For this review, take the finished solid that the model builds, in its own axes (mm). Face numbers are marked on the shaded views. A direction names the side the tool comes from. Give positions to 0.01 mm unless a question says otherwise; leave off trailing zeros. Order: outer loops, then holes, each group sorted by start corner. A loop starts at its lowest first (then second) coordinate and runs counter-clockwise, first axis right, second up.
Item 1: Consider section B-B (z = 28.03). Give the boundary of the cut face in (x, y), plus the area to 3 significant figures.
Item 2: The part is to be moulded in two halves that separate along X. For the marked faces 1, 2 and 3, say which applies: released by +X, released by -X, zero draft, split by the parting line, or undercut.
Item 3: For probe 1 along X at (y, z) = (22, -1); probe 2 along X at (y, z) = (29.45, -28.03); probe 3 along Y at (x, z) = (65, -21.5), list the stretches that pass through material, from the lowest coordinate up.
Item 4: For P1, Ø8, axis at x = 50, y = 24.5, coming from the -Z side; P2, Ø3, axis at x = 160.22, z = -15.57, coming from the +Y side; P3, Ø12, axis at x = 166, z = 5, coming from the +Y side; P4, Ø3, axis at x = -41.22, z = 0, coming from the +Y side, all flat-tipped, find the tip position at first contact; note any pin that passes through.
Item 5: Machinability: for the marked faces 4, 5 and 6, which of the approach directions +Z, -Z, +X, -X, +Y, -Y give a long, thin tool a straight path to every point of the face, cutting with its end or side? Answer none if there is none.
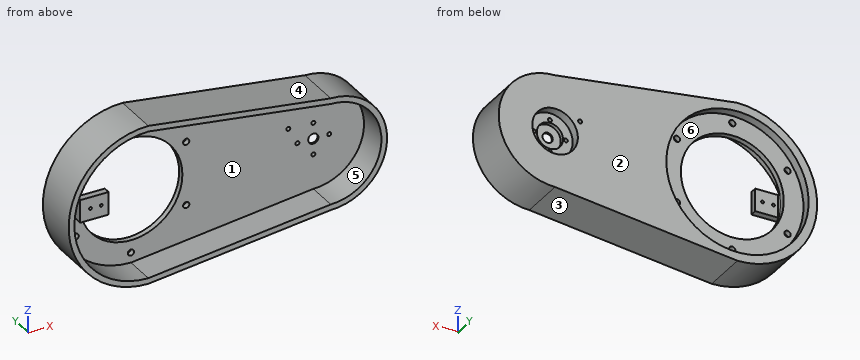
```python
from build123d import *

# Parameters (mm, degrees)
BOSS_EXTRUDE1_DEPTH = 40
SKETCH2_R           = 45.22
SKETCH2_R_2         = 2.75
CUT_EXTRUDE1_DEPTH  = 28
SKETCH4_R           = 62.5
CUT_EXTRUDE2_DEPTH  = 8
CUT_EXTRUDE3_DEPTH  = 27
SKETCH6_R           = 4.5
SKETCH6_R_2         = 1.75
CUT_EXTRUDE4_DEPTH  = 23
SKETCH6_3_R         = 11.5
SKETCH6_3_R_2       = 4.5
CUT_EXTRUDE5_DEPTH  = 11.5
BOSS_EXTRUDE2_DEPTH = 10
SKETCH8_W           = 20
SKETCH8_H           = 6
BOSS_EXTRUDE3_DEPTH = 20
SKETCH9_R           = 1.25
CUT_EXTRUDE6_DEPTH  = 20
SKETCH6_4_R         = 20
CUT_EXTRUDE7_DEPTH  = 8
SKETCH11_R          = 4.5
SKETCH11_R_2        = 1.75
CUT_EXTRUDE8_DEPTH  = 168


with BuildPart() as part:
    # Sketch1 → Boss-Extrude1 (new body)
    with BuildSketch(Plane(origin=(0, 0, 0), x_dir=(1, 0, 0), z_dir=(0, 1, 0))):
        with BuildLine():
            Line((0, 70), (160.2226, 51.102080384))
            ThreePointArc((160.2226, 51.102080384), (209.74985375, 1.574826635), (160.2226, -47.952427115))
            Line((160.2226, -47.952427115), (0, -70))
            ThreePointArc((0, -70), (-70, 0), (0, 70))
        make_face()
    extrude(amount=BOSS_EXTRUDE1_DEPTH)

    # Sketch2 → Cut-Extrude1 (cut)
    with BuildSketch(Plane(origin=(0, 40, 0), x_dir=(1, 0, 0), z_dir=(0, 1, 0))):
        Circle(SKETCH2_R)
        with Locations((0, 56.06)):
            Circle(SKETCH2_R_2)
        with Locations((-48.549384136, 28.03)):
            Circle(SKETCH2_R_2)
        with Locations((-48.549384136, -28.03)):
            Circle(SKETCH2_R_2)
        with Locations((0, -56.06)):
            Circle(SKETCH2_R_2)
        with Locations((48.549384136, -28.03)):
            Circle(SKETCH2_R_2)
        with Locations((48.549384136, 28.03)):
            Circle(SKETCH2_R_2)
    extrude(amount=-CUT_EXTRUDE1_DEPTH, mode=Mode.SUBTRACT)

    # Sketch4 → Cut-Extrude2 (cut)
    with BuildSketch(Plane(origin=(0, 40, 0), x_dir=(1, 0, 0), z_dir=(0, 1, 0))):
        Circle(SKETCH4_R)
    extrude(amount=-CUT_EXTRUDE2_DEPTH, mode=Mode.SUBTRACT)

    # Sketch5 → Cut-Extrude3 (cut)
    with BuildSketch(Plane.XZ):
        with BuildLine():
            Line((160.2226, 42.955173365), (0, 65))
            ThreePointArc((0, 65), (-65, 0), (0, -65))
            Line((0, -65), (160.2226, -46.104826635))
            ThreePointArc((160.2226, -46.104826635), (204.7526, -1.574826635), (160.2226, 42.955173365))
        make_face()
    extrude(amount=-CUT_EXTRUDE3_DEPTH, mode=Mode.SUBTRACT)

    # Sketch6 → Cut-Extrude4 (cut)
    with BuildSketch(Plane(origin=(0, 40, 0), x_dir=(1, 0, 0), z_dir=(0, 1, 0))):
        with Locations((160.2226, 1.574826635)):
            Circle(SKETCH6_R)
        with Locations((160.2226, -12.425173365)):
            Circle(SKETCH6_R_2)
        with Locations((174.2226, 1.574826635)):
            Circle(SKETCH6_R_2)
        with Locations((160.2226, 15.574826635)):
            Circle(SKETCH6_R_2)
        with Locations((146.2226, 1.574826635)):
            Circle(SKETCH6_R_2)
    extrude(amount=-CUT_EXTRUDE4_DEPTH, mode=Mode.SUBTRACT)

    # Sketch6_3 → Cut-Extrude5 (cut)
    with BuildSketch(Plane(origin=(0, 40, 0), x_dir=(1, 0, 0), z_dir=(0, 1, 0))):
        with Locations((160.2226, 1.574826635)):
            Circle(SKETCH6_3_R)
        with Locations((160.2226, 1.574826635)):
            Circle(SKETCH6_3_R_2, mode=Mode.SUBTRACT)
    extrude(amount=-CUT_EXTRUDE5_DEPTH, mode=Mode.SUBTRACT)

    # Sketch7 → Boss-Extrude2 (add)
    with BuildSketch(Plane.XZ.offset(-27)):
        Polygon((-45.22, 0), (-45.22, 10), (-50.22, 10), (-50.22, -10), (-45.22, -10), align=None)
    extrude(amount=BOSS_EXTRUDE2_DEPTH)

    # Sketch8 → Boss-Extrude3 (add)
    with BuildSketch(Plane(origin=(-45.22, 0, 0), x_dir=(0, 0, -1), z_dir=(1, 0, 0))):
        with Locations((0, 20)):
            Rectangle(SKETCH8_W, SKETCH8_H)
    extrude(amount=BOSS_EXTRUDE3_DEPTH)

    # Sketch9 → Cut-Extrude6 (cut)
    with BuildSketch(Plane.XZ.offset(-17)):
        with Locations((-31.72, 0)):
            Circle(SKETCH9_R)
        with Locations((-41.22, 0)):
            Circle(SKETCH9_R)
    extrude(amount=-CUT_EXTRUDE6_DEPTH, mode=Mode.SUBTRACT)

    # Sketch6_4 → Cut-Extrude7 (cut)
    with BuildSketch(Plane(origin=(0, 40, 0), x_dir=(1, 0, 0), z_dir=(0, 1, 0))):
        with Locations((160.2226, 1.574826635)):
            Circle(SKETCH6_4_R)
    extrude(amount=-CUT_EXTRUDE7_DEPTH, mode=Mode.SUBTRACT)

    # Sketch11 → Cut-Extrude8 (cut)
    with BuildSketch(Plane.XZ.offset(-27)):
        with Locations((160.2226, -1.574826635)):
            Circle(SKETCH11_R)
        with Locations((138.2226, 13.425173365)):
            Circle(SKETCH11_R_2)
    extrude(amount=-CUT_EXTRUDE8_DEPTH, mode=Mode.SUBTRACT)


solid = part.part
```
Resolved:
1. outline: (-64.14, 0) - (-58.65, 0) - (-58.65, 27) - (-51.3, 27) - (-51.3, 32) - (-55.86, 32) - (-55.86, 40) - (-64.14, 40) - close; (-45.8, 27) - (-35.48, 27) - (-35.48, 32) - (-45.8, 32) - close; (35.48, 27) - (45.8, 27) - (45.8, 32) - (35.48, 32) - close; (51.3, 27) - (193.49, 27) - (193.49, 0) - (199.93, 0) - (199.93, 40) - (55.86, 40) - (55.86, 32) - (51.3, 32) - close
1. area: 2,450 mm2
2. face 1: undercut
2. face 2: zero draft
2. face 3: released by +X
3. probe 1: x = -69.99 to -64.99, -50.22 to -41.97, -40.47 to -32.47, -30.97 to -25.22, 204.75 to 209.75
3. probe 2: x = -64.14 to -51.3, -45.8 to -35.48, 35.48 to 45.8, 51.3 to 202.09
3. probe 3: y = 27 to 40
4. P1: stops at z = -64.57
4. P2: passes through
4. P3: stops at y = 32
4. P4: stops at y = 23
5. face 4: +Z, +X, +Y, -Y
5. face 5: -Y
5. face 6: +Y
